Autodesk Inventor part; units mm, degrees
ref_plane "YZ Plane" through (0, 0, 0) normal (1, 0, 0) x (0, 1, 0)
ref_plane "XZ Plane" through (0, 0, 0) normal (0, 1, 0) x (-1, 0, 0)
ref_plane "XY Plane" through (0, 0, 0) normal (0, 0, 1) x (1, 0, 0)
sketch "Sketch1" plane through (0, 0, 0) normal (0, 0, 1) x (1, 0, 0)
  circle A0 centre (0, 0) radius 3.8862
  dimension "d0" = 7.7724
extrude "Extrusion1" add sketch "Sketch1" along normal blind 16.9672
sketch "Sketch2" plane through (0, 0, 16.9672) normal (0, 0, 1) x (1, 0, 0)
  circle A0 centre (0, 0) radius 3.8862
  circle A1 centre (0, 0) radius 3.5
  dimension "d4" = 7
extrude "Extrusion2" add sketch "Sketch2" along normal blind 5.0328 contours A1
sketch "Sketch3" plane through (0, 0, 22) normal (0, 0, 1) x (1, 0, 0)
  circle A0 centre (0, 0) radius 3.5
  circle A1 centre (0, 0) radius 10
  dimension "d8" = 20
extrude "Extrusion3" add sketch "Sketch3" along normal blind 5.94 contours A0 | A1
sketch "Sketch4" plane through (0, 0, 27.94) normal (0, 0, 1) x (1, 0, 0)
  circle A0 centre (0, 0) radius 10
  circle A1 centre (0, 0) radius 3.75
  dimension "d13" = 7.5
extrude "Extrusion4" add sketch "Sketch4" along normal blind 1.1 contours A1
sketch "Sketch5" plane through (0, 0, 29.04) normal (0, 0, 1) x (1, 0, 0)
  circle A0 centre (0, 0) radius 3.75
  circle A1 centre (0, 0) radius 1.4605
  dimension "d18" = 2.921
extrude "Extrusion5" cut sketch "Sketch5" against normal up to next contours A1
properties part number "stator"
Model file for the job. Use its own axes, mm. A direction names the side the tool comes from. Coordinates: 2 decimals unless noted, no trailing zeros. Loops run counter-clockwise (first coordinate to the right, second up) from the corner with the lowest first, then second, coordinate; pieces in that order, holes last. Notation, with made-up numbers: (1, 13) -> (56, 13) arc R23 ccw to (56, 33) -> close; hole circle Ø3 at (-26, -33.75). An arc over 180 degrees is marked (long way). Use one line per item in the form item = value. Start each with the question number.
(1) Probe probe 1 along Y at (x, z) = (0, 7.5); probe 2 along Z at (x, y) = (1, 5.25); probe 3 along Y at (x, z) = (0, 23.25). List the from-to ranges inside material, lowest first. Write a range as from..to.
(2) Pull direction Z, two halves, no side cores. Call faces 1 (the flat face through (4, 0, 27.94)), 2 (the cylindrical face through (-2.17, 9.76, 24.93)), 3 (the cylindrical face through (3.233, 1.341, 19.448)), 4 (the flat face through (2, 0, 0)): pulls with the +Z half, pulls with the -Z half, needs draft (parallel to the pull), parting line crosses it, or undercut.
(3) Tool access for faces 5 (the cylindrical face through (-3.746, -0.165, 28.482)), 6 (the flat face through (0, -2, 29.04)), 7 (the cylindrical face through (3.707, -1.167, 8.365)): list every direction of +Z, -Z, +X, -X, +Y, -Y with a clear straight run to the whole face (end or side of a thin tool).
(4) Cut at D-D on z = 8.5. Give the cut face in (x, y), and give its area (3 significant figures).
(5) Flat gauge pins, fed straight in: pin 1 (10 mm diameter, centred on y = -5.5, z = 7, fed in from +X); pin 2 (1 mm diameter, centred on x = -4.5, y = 5, fed in from -Z); pin 3 (1 mm diameter, centred on x = -3.5, z = 19.5, fed in from +Y). Where does each tip first touch, or does it go through?
(6) Cut at A-A on x = 0. Give the cut face in (y, z).
(7) Cut at C-C on y = -2.25. Give the cut face in (x, z), and give its area (3 significant figures).
Values:
q1.probe_1 = -3.89..-1.46, 1.46..3.89
q1.probe_2 = 22..27.94
q1.probe_3 = -10..-1.46, 1.46..10
q2.face_1 = pulls with the +Z half
q2.face_2 = needs draft
q2.face_3 = undercut
q2.face_4 = pulls with the -Z half
q3.face_5 = +Z
q3.face_6 = +Z, +X, -X, +Y, -Y
q3.face_7 = -Z
q4.outline = circle Ø7.77 at (0, 0); hole circle Ø2.92 at (0, 0)
q4.area = 40.7 mm2
q5.pin_1 = 3.85
q5.pin_2 = 22
q5.pin_3 = 1.8
q6.outline = (-10, 22) -> (-3.5, 22) -> (-3.5, 16.97) -> (-3.89, 16.97) -> (-3.89, 0) -> (-1.46, 0) -> (-1.46, 29.04) -> (-3.75, 29.04) -> (-3.75, 27.94) -> (-10, 27.94) -> close; (1.46, 0) -> (3.89, 0) -> (3.89, 16.97) -> (3.5, 16.97) -> (3.5, 22) -> (10, 22) -> (10, 27.94) -> (3.75, 27.94) -> (3.75, 29.04) -> (1.46, 29.04) -> close
q7.outline = (-9.74, 22) -> (-2.68, 22) -> (-2.68, 16.97) -> (-3.17, 16.97) -> (-3.17, 0) -> (3.17, 0) -> (3.17, 16.97) -> (2.68, 16.97) -> (2.68, 22) -> (9.74, 22) -> (9.74, 27.94) -> (3, 27.94) -> (3, 29.04) -> (-3, 29.04) -> (-3, 27.94) -> (-9.74, 27.94) -> close
q7.area = 257 mm2
